```python
from build123d import *

# Parameters (mm, degrees)
F0_W     = 60
F0_H     = 20
F0_W_2   = 20
F0_H_2   = 60
F0_W_3   = 40
F1_DEPTH = 5
F2_R     = 1.8
F3_DEPTH = 26
F4_R     = 1.8
F5_DEPTH = 20


with BuildPart() as f1:
    # F0 (on Top) → F1 (new body, symmetric)
    with BuildSketch(Plane.XY):
        with Locations((-138.214068, 3.086677)):
            Rectangle(F0_W, F0_H)
        with BuildLine():
            ThreePointArc((-98.142568, 19.663455), (-102.199728, 14.87648), (-108.214068, 13.086677))
            Line((-108.214068, 13.086677), (-108.214068, -6.913323))
            ThreePointArc((-108.214068, -6.913323), (-87.188123, -0.402812), (-78.142568, 19.663455))
            Line((-78.142568, 19.663455), (-98.142568, 19.663455))
        make_face()
        with Locations((-88.142568, 49.663455)):
            Rectangle(F0_W_2, F0_H_2)
        with BuildLine():
            ThreePointArc((-102.141655, 83.454146), (-99.386567, 82.355881), (-98.142568, 79.663455))
            Line((-98.142568, 79.663455), (-78.142568, 79.663455))
            ThreePointArc((-78.142568, 79.663455), (-85.245257, 96.49855), (-102.141655, 103.454146))
            Line((-102.141655, 103.454146), (-102.141655, 83.454146))
        make_face()
        with Locations((-122.141655, 93.454146)):
            Rectangle(F0_W_3, F0_H)
        Polygon((-149.557854, 86.454146), (-142.141655, 83.454146), (-142.141655, 103.454146), (-149.557854, 100.454146), align=None)
    extrude(amount=F1_DEPTH, both=True)

    # F2 (on face) → F3 (cut)
    with BuildSketch(Plane.XY.offset(5)):
        with Locations((-157.338008, 3.086677)):
            Circle(F2_R)
    extrude(amount=-F3_DEPTH, mode=Mode.SUBTRACT)

    # F4 (on face) → F5 (cut)
    with BuildSketch(Plane.XY.offset(5)):
        with Locations((-102.756642, 3.086677)):
            Circle(F4_R)
    extrude(amount=-F5_DEPTH, mode=Mode.SUBTRACT)


solid = f1.part
```
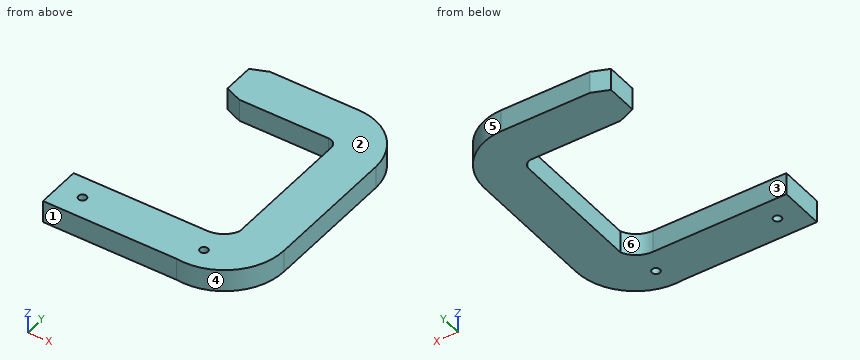
Geometry check sheet. Reference: the model listing, model coordinates, mm. Face numbers are marked on the shaded views. A direction names the side the tool comes from. Give positions to 0.01 mm unless a question says otherwise; leave off trailing zeros. Order: outer loops, then holes, each group sorted by start corner. A loop starts at its lowest first (then second) coordinate and runs counter-clockwise, first axis right, second up. Notation, with made-up numbers: (69, 63.25) - (126, 63.25) arc R27 cw to (126, 96.25) - close; hole circle Ø6 at (-8, 30). An arc over 180 degrees is marked (long way). Write item = value, one per line. Start each with the question number.
1) Draft check along Y on the marked faces 4, 5 and 6. Enter one of: released by +Y, released by -Y, zero draft, split by the parting line, or undercut.
2) Access from +Z, -Z, +X, -X, +Y, -Y to the whole of each face (thin tool, end or side, straight path). Record for the marked faces 1, 2 and 3.
3) Gauge pin test, flat ends, axial feed: pin 1 Ø5 at (y, z) = (96, 1) entering from -X; pin 2 Ø2 at (x, z) = (-121, -0.5) entering from -Y; pin 3 Ø3 at (y, z) = (52, 0.5) entering from -X. Record the tip position at first contact, or that the pin passes through.
4) Scan lines: L1, parallel to Y at x = -112.5, z = 0.5; L2, parallel to X at y = 40.5, z = -1.5; L3, parallel to Y at x = -162, z = -3.5. Record each from-to range of solid material in increasing order.
5) Section check B-B (z = 0.75). Enter the section's corners in (x, y).
6) Section check C-C (x = -151). Enter the section's corners in (y, z).
7) Section check D-D (y = 39). Enter the section's corners in (x, z), then the cut area to 3 significant figures.
8) Section check A-A (x = -135.5). Enter the section's corners in (y, z).
Geometry check:
q1.face_4 = released by -Y
q1.face_5 = released by +Y
q1.face_6 = undercut
q2.face_1 = +Z, -Z, -X, -Y
q2.face_2 = +Z, +X, -X, +Y, -Y
q2.face_3 = +Z, -Z, -X
q3.pin_1 = -149.56
q3.pin_2 = -6.91
q3.pin_3 = -98.14
q4.L1 = -6.91 to 13.09, 83.45 to 103.45
q4.L2 = -98.14 to -78.14
q4.L3 = -6.91 to 13.09
q5.outline = (-168.21, -6.91) - (-108.21, -6.91) arc R26.78 ccw to (-78.14, 19.66) - (-78.14, 79.66) arc R24 ccw to (-102.14, 103.45) - (-142.14, 103.45) - (-149.56, 100.45) - (-149.56, 86.45) - (-142.14, 83.45) - (-102.14, 83.45) arc R4 cw to (-98.14, 79.66) - (-98.14, 19.66) arc R11 cw to (-108.21, 13.09) - (-168.21, 13.09) - close; hole circle Ø3.6 at (-157.34, 3.09); hole circle Ø3.6 at (-102.76, 3.09)
q6.outline = (-6.91, -5) - (13.09, -5) - (13.09, 5) - (-6.91, 5) - close
q7.outline = (-98.14, -5) - (-78.14, -5) - (-78.14, 5) - (-98.14, 5) - close
q7.area = 200 mm2
q8.outline = (-6.91, -5) - (13.09, -5) - (13.09, 5) - (-6.91, 5) - close; (83.45, -5) - (103.45, -5) - (103.45, 5) - (83.45, 5) - close
